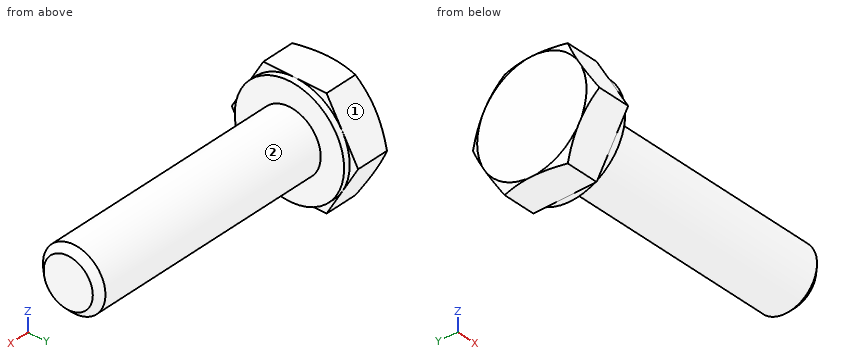
Autodesk Inventor part; units mm, degrees
ref_plane "Work Plane1" through (1.525, 0, 0) normal (0, 0, 1) x (1, 0, 0)
ref_plane "YZ Plane" through (0, 0, 0) normal (1, 0, 0) x (0, 1, 0)
ref_plane "XZ Plane" through (0, 0, 0) normal (0, 1, 0) x (-1, 0, 0)
sketch "Sketch1" plane through (0, 0, 0) normal (0, 0, 1) x (1, 0, 0)
  line L0 (0, 3.5) -> (0, 2)
  line L1 (2.1, 2) -> (16, 2)
  line L2 (16, 2) -> (16, 0)
  line L3 (16, 0) -> (-0.4001, 0)
  line L4 (-3.6801, 0) -> (19.28, 0)
  line L5 (-0.4001, 0) -> (-0.4001, 3.5)
  line L6 (-0.4001, 3.5) -> (0, 3.5)
  line L7 (2.1, 2) -> (1.6705, 2)
  line L8 (1.6705, 2) -> (0, 2)
  line L9 (0, -0.7) -> (0, 4.2)
  dimension "d0" = 16
  dimension "d1" = 13.9
  dimension "d2" = 4
  dimension "d9" = 0.4001
  dimension "d10" = 7
  dimension "d13" = 0.4295
  dimension "d14" = 4
revolve "Body" add sketch "Sketch1" angle 360 about axis through (16, 0, 0) along (-1, 0, 0)
sketch "Sketch2" plane through (-0.4001, 0, 0) normal (-1, 0, 0) x (0, 0, 1)
  line L0 (0, 4.0415) -> (3.5, 2.0207)
  line L1 (3.5, 2.0207) -> (3.5, -2.0207)
  line L2 (3.5, -2.0207) -> (0, -4.0415)
  line L3 (0, -4.0415) -> (-3.5, -2.0207)
  line L4 (-3.5, -2.0207) -> (-3.5, 2.0207)
  line L5 (-3.5, 2.0207) -> (0, 4.0415)
  point P0 (0, 0)
  point P1 (0, 0)
  dimension "d11" = 7
extrude "Head" add sketch "Sketch2" along normal blind 2.4
sketch "Sketch4" plane through (0, 0, 0) normal (0, 0, 1) x (1, 0, 0)
  line L0 (-2.8001, 3.5) -> (-2.8001, 4.0415)
  line L1 (-2.8001, 4.0415) -> (-2.4875, 4.0415)
  line L2 (-2.4875, 4.0415) -> (-2.8001, 3.5)
  line L3 (-3.2801, 0) -> (0.0799, 0)
  line L4 (-0.4001, 4.0415) -> (-2.8001, 4.0415)
  line L5 (-2.8001, 2.0207) -> (-2.8001, 4.0415)
  dimension "d5" = 30
  dimension "d19" = 7
revolve "Chamfer1" cut sketch "Sketch4" angle 360 about axis through (-10, 0, 0) along (1, 0, 0)
thread "Thread"
chamfer "Chamfer2" distance 0.4294 distance2 0.4295 1 edges at (16, -2, 0) measured on face at (16, 0.6473, -0.1595)
ref_plane "Work Plane1" through (1.525, 0, 0) normal (0, 0, 1) x (1, 0, 0)
equation "\"d0\" = NLG"
equation "\"d1\" = GEL"
equation "\"d2\" = GD"
equation "\"d10\" = SD2"
equation "\"d14\" = BDM"
equation "\"d11\" = SW"
equation "\"d3\" = KOH - SD"
equation "\"d5\" = ANG1"
equation "\"d19\" = SW0"
equation "\"d15\" = GEL"
equation "\"d6\" = -0.5 * SPD + 0.5 * GD"
equation "\"NLG\" = 16"
equation "\"GD\" = NND"
equation "\"BDM\" = NND"
equation "\"KOH\" = 2.8"
equation "\"GEL\" = 13.9"
equation "\"SW\" = 7"
equation "\"SW0\" = SW"
equation "\"SPD\" = NND - 1.2269 * PTC"
equation "\"SD2\" = SW"
equation "\"SD\" = 0.4"
equation "\"ANG1\" = 30deg"
equation "\"GAL\" = 0.61345 * PTC"
equation "\"GUL\" = 0.61345 * PTC"
equation "\"RR\" = 0.2"
equation "\"WFT\" = SD"
equation "\"GD1\" = THREADDIA - 1.2269 * PTC"
equation "\"THREADDIA\" = 4"
equation "\"SDH\" = SW"
equation "\"TOA\" = 30deg"
equation "\"FAWI\" = 45deg"
equation "\"PTC\" = 0.7"
equation "\"NND\" = 4"
equation "\"E0\" = 1.155 * SW"
properties part number "AS 1110 - M4 x 16" material "Steel, Mild"
Geometry: final body of the model. Coordinates: model frame, mm. Face numbers are marked on the shaded views. A direction names the side the tool comes from. Give positions to 0.01 mm unless a question says otherwise; leave off trailing zeros. Order: outer loops, then holes, each group sorted by start corner. A loop starts at its lowest first (then second) coordinate and runs counter-clockwise, first axis right, second up. Notation, with made-up numbers: M 22.25,69.5 L 47.25,69.5 A8 ccw 47.25,75.5 Z; hole C 71,-17 d10. An arc over 180 degrees is marked long. Answer as CSV lines item,"result". Start each with the question number.
1) Set-up query: the marked faces 1 and 2. Return all of +Z, -Z, +X, -X, +Y, -Y with unobstructed straight access to the full face (end or side cutting, diameter ignored); none if empty.
2) Cut plane A-A (x = 1.25). Output: boundary loops of the cut face in (y, z), then the cut area to 3 significant figures.
3) First-contact query: P1, Ø1.9, axis at y = 1, z = 3, coming from the +X side; P2, Ø4, axis at x = 6, z = -0.5, coming from the -Y side; P3, Ø1.5, axis at x = 0.5, y = -1, coming from the +Z side. Flat tips, straight axial feed; report the tip coordinate or a pass-through.
4) Line query: line 1 (X direction, y = 0.25, z = 2.25); line 2 (Z direction, x = 0.25, y = -0.75); line 3 (Y direction, x = 6, z = 1.25). Output: solid intervals per line, ascending. Write a range as from..to.
Findings below:
1,face 1,"+Z, +X, -X, +Y"
1,face 2,"+X"
2,outline,"C 0,0 d4"
2,area,"12.6 mm²"
3,P1,"stops at x = 0"
3,P2,"stops at y = -2"
3,P3,"stops at z = 3.47"
4,line 1,"x = -2.8..0"
4,line 2,"z = -1.85..1.85"
4,line 3,"y = -1.56..1.56"
